from build123d import *

# Parameters (mm, degrees)
PAD_DEPTH        = 4
POCKET_DEPTH     = 1.5
SKETCH003_R      = 2
PAD001_DEPTH     = 7
HOLE_D           = 4.3
HOLE_DEPTH       = 25
HOLE_CSINK_D     = 8
HOLE_CSINK_ANGLE = 90


with BuildPart() as part:
    # Sketch → Pad (new body)
    with BuildSketch(Plane.XY):
        with BuildLine():
            ThreePointArc((12.057778, 7.5), (-14.2, 0), (12.057778, -7.5))
            Line((15, -7.5), (12.057778, -7.5))
            Line((15, -25), (15, -7.5))
            Line((-15, -25), (15, -25))
            Line((-15, 25), (-15, -25))
            Line((15, 25), (-15, 25))
            Line((15, 7.5), (15, 25))
            Line((12.057778, 7.5), (15, 7.5))
        make_face()
    extrude(amount=PAD_DEPTH)

    # Sketch002 → Pocket (cut)
    with BuildSketch(Plane.XY.offset(4)):
        with BuildLine():
            ThreePointArc((3.6, 17.5), (0, 21.1), (-3.6, 17.5))
            Line((-3.6, 17.5), (-3.6, -17.5))
            ThreePointArc((-3.6, -17.5), (0, -21.1), (3.6, -17.5))
            Line((3.6, -17.5), (3.6, 17.5))
        make_face()
    extrude(amount=-POCKET_DEPTH, mode=Mode.SUBTRACT)

    # Sketch003 → Pad001 (join)
    with BuildSketch(Plane.XY):
        with Locations((0, 17.5)):
            Circle(SKETCH003_R)
        with Locations((0, -17.5)):
            Circle(SKETCH003_R)
    extrude(amount=PAD001_DEPTH)

    # Hole
    with Locations(Plane(origin=(0, 0, 0), x_dir=(1, 0, 0), z_dir=(0, 0, -1))):
        with Locations((-10, -20), (10, -20), (10, 20), (-10, 20)):
            CounterSinkHole(HOLE_D / 2, HOLE_CSINK_D / 2, depth=HOLE_DEPTH, counter_sink_angle=HOLE_CSINK_ANGLE)


solid = part.part
Could you check a few things on this model? Use its own coordinates, in mm. A direction names the side the tool comes from. Give positions to 0.01 mm unless a question says otherwise; leave off trailing zeros. Order: outer loops, then holes, each group sorted by start corner. A loop starts at its lowest first (then second) coordinate and runs counter-clockwise, first axis right, second up.
Item 1: If we mould it in two halves opening along X, with no side actions, what happens to faces 4 (the face through (15, -16, 2)), 5 (the face through (0, -17, 7)), 6 (the face through (3.6, 16, 3))? For each: pulls with the +X half, pulls with the -X half, needs draft (parallel to the pull), parting line crosses it, or undercut.
Item 2: If we section it at C-C, the plane z = 4.5: Write out the boundary of the cut face in (x, y).
Item 3: If we section it at A-A, the plane x = 0: Write out the boundary of the cut face in (y, z), plus the area to 3 significant figures.
Item 4: If we section it at B-B, the plane y = 20: Write out the boundary of the cut face in (x, z), plus the area to 3 significant figures.
Item 5: I'm going to push flat-ended pins straight in: pin 1 (4 mm diameter, centred on x = -10, y = 20, fed in from +Z); pin 2 (5 mm diameter, centred on x = -6.5, y = 13.5, fed in from +Z). Where does each tip first touch, or does it pass through?
Item 6: I need wall thicknesses on line 1 (Y direction, x = 1.25, z = 3.5); line 2 (Y direction, x = 0, z = 2.35); line 3 (X direction, y = 20, z = 2.75). Which ranges of each line are inside material? Lowest first, please.
Item 7: If we section it at D-D, the plane x = -10: Write out the boundary of the cut face in (y, z).
Item 8: For faces 1 (the face through (-0.1, -21.1, 3.3)), 2 (the face through (0, 25, 2)), 3 (the face through (14, 7.5, 2)), which set-ups out of +Z, -Z, +X, -X, +Y, -Y let a thin tool reach every point of the face, with its end or its side?
Values:
1. face 4: pulls with the +X half
1. face 5: needs draft
1. face 6: undercut
2. outline: circle Ø4 at (0, -17.5); circle Ø4 at (0, 17.5)
3. outline: (-25, 0) - (-14.2, 0) - (-14.2, 2.5) - (-15.5, 2.5) - (-15.5, 7) - (-19.5, 7) - (-19.5, 2.5) - (-21.1, 2.5) - (-21.1, 4) - (-25, 4) - close; (14.2, 0) - (25, 0) - (25, 4) - (21.1, 4) - (21.1, 2.5) - (19.5, 2.5) - (19.5, 7) - (15.5, 7) - (15.5, 2.5) - (14.2, 2.5) - close
3. area: 102 mm2
4. outline: (-15, 0) - (-14, 0) - (-12.15, 1.85) - (-12.15, 4) - (-15, 4) - close; (-7.85, 1.85) - (-6, 0) - (6, 0) - (7.85, 1.85) - (7.85, 4) - (2.59, 4) - (2.59, 2.5) - (-2.59, 2.5) - (-2.59, 4) - (-7.85, 4) - close; (12.15, 1.85) - (14, 0) - (15, 0) - (15, 4) - (12.15, 4) - close
4. area: 71.0 mm2
5. pin 1: passes through
5. pin 2: stops at z = 4
6. line 1: y = -25 to -20.88, -19.06 to -15.94, 15.94 to 19.06, 20.88 to 25
6. line 2: y = -25 to -14.2, 14.2 to 25
6. line 3: x = -15 to -12.15, -7.85 to -2.59, 2.59 to 7.85, 12.15 to 15
7. outline: (-25, 0) - (-24, 0) - (-22.15, 1.85) - (-22.15, 4) - (-25, 4) - close; (-17.85, 1.85) - (-16, 0) - (-10.08, 0) - (-10.08, 4) - (-17.85, 4) - close; (10.08, 0) - (16, 0) - (17.85, 1.85) - (17.85, 4) - (10.08, 4) - close; (22.15, 1.85) - (24, 0) - (25, 0) - (25, 4) - (22.15, 4) - close
8. face 1: +Z
8. face 2: +Z, -Z, +X, -X, +Y
8. face 3: +Z, -Z, +X
